```python
from build123d import *

# Parameters (mm, degrees)
BOSS_EXTRUDE1_DEPTH = 6
FILLET1_R           = 2
SKETCH2_R           = 1.5
CUT_EXTRUDE1_DEPTH  = 10
SKETCH3_W           = 6
SKETCH3_H           = 18.774257397
BOSS_EXTRUDE2_DEPTH = 2
FILLET2_R           = 10
SKETCH4_W           = 6
SKETCH4_H           = 2
BOSS_EXTRUDE3_DEPTH = 5
SKETCH5_W           = 6
SKETCH5_H           = 2
BOSS_EXTRUDE4_DEPTH = 7


with BuildPart() as part:
    # Sketch1 → Boss-Extrude1 (new body)
    with BuildSketch(Plane.XY):
        with BuildLine():
            Line((4.974937186, 0.5), (9.527119886, 0.5))
            Line((9.527119886, 0.5), (60, 0.5))
            Line((60, 0.5), (60, -40.25))
            Line((60, -40.25), (62, -40.25))
            Line((62, -40.25), (62, 4.331195296))
            Line((62, 4.331195296), (60, 4.331195296))
            Line((60, 4.331195296), (60, 2.5))
            Line((60, 2.5), (5.454356057, 2.5))
            ThreePointArc((5.454356057, 2.5), (-6, 0), (5.454356057, -2.5))
            Line((5.454356057, -2.5), (20, -2.5))
            Line((20, -2.5), (20, -0.5))
            Line((20, -0.5), (4.974937186, -0.5))
            Line((4.974937186, -0.5), (3.968626967, -0.5))
            ThreePointArc((3.968626967, -0.5), (-4, 0), (3.968626967, 0.5))
            Line((3.968626967, 0.5), (4.974937186, 0.5))
        make_face()
    extrude(amount=BOSS_EXTRUDE1_DEPTH)

    # Fillet1
    # the kernel refuses this fillet: 2 mm, written as the material it adds along each edge
    with BuildSketch(Plane(origin=(5.454356057, -2.5, 0), x_dir=(1, 0, 0), z_dir=(0, 0, 1))) as fillet1_piece_1:
        with BuildLine():
            CenterArc((1.16002222, -2), FILLET1_R, 90, 55.771133672)
            Line((-0.493572349, -0.875), (-0.52664424, -0.8525))
            ThreePointArc((-0.52664424, -0.8525), (-0.26328023, -0.428195989), (-0.036362374, 0.016666667))
            Line((-0.036362374, 0.016666667), (0, 0.04))
            Line((0, 0.04), (1.16002222, 0.04))
            Line((1.16002222, 0.04), (1.16002222, 0))
        make_face()
    extrude(amount=6)
    with BuildSketch(Plane(origin=(5.454356057, 2.5, 0), x_dir=(-0.491308051869414, 0.8709858771348026, 0), z_dir=(0, 0, 1))) as fillet1_piece_2:
        with BuildLine():
            CenterArc((1.172043497, -1.992979075), FILLET1_R, 94.802273988, 55.771133672)
            Line((-0.569928257, -1.010362971), (-0.604767692, -0.990710649))
            Line((-0.604767692, -0.990710649), (-0.034839435, 0.019652322))
            Line((-0.034839435, 0.019652322), (0.003348696, 0.039859581))
            ThreePointArc((0.003348696, 0.039859581), (0.502304356, 0.018937224), (1.001260016, 0.039859581))
            Line((1.001260016, 0.039859581), (1.004608712, 0))
        make_face()
    extrude(amount=6)
    with BuildSketch(Plane(origin=(60, 2.5, 0), x_dir=(-1, 0, 0), z_dir=(0, 0, 1))) as fillet1_piece_3:
        with BuildLine():
            CenterArc((1.992863511, -2), FILLET1_R, 90, 85.158341327)
            Line((0, -1.831195296), (-0.03985727, -1.827819202))
            ThreePointArc((-0.03985727, -1.827819202), (-0.04, -0.915597648), (-0.04, 0))
            Line((-0.04, 0), (0, 0.04))
            Line((0, 0.04), (1.992863511, 0.04))
            Line((1.992863511, 0.04), (1.992863511, 0))
        make_face()
    extrude(amount=6)
    with BuildSketch(Plane(origin=(60, 0.5, 0), x_dir=(-1, 0, 0), z_dir=(0, 0, 1))) as fillet1_piece_4:
        with BuildLine():
            CenterArc((FILLET1_R, FILLET1_R), FILLET1_R, 180, 90)
            Line((0, FILLET1_R), (-FILLET1_R * 0.02, FILLET1_R))
            Line((-FILLET1_R * 0.02, FILLET1_R), (-FILLET1_R * 0.02, -FILLET1_R * 0.02))
            Line((-FILLET1_R * 0.02, -FILLET1_R * 0.02), (FILLET1_R, -FILLET1_R * 0.02))
            Line((FILLET1_R, -FILLET1_R * 0.02), (FILLET1_R, 0))
        make_face()
    extrude(amount=6)

    # Sketch2 → Cut-Extrude1 (cut)
    with BuildSketch(Plane.XZ.offset(2.5)):
        with Locations((13.307189139, 3)):
            Circle(SKETCH2_R)
    extrude(amount=-CUT_EXTRUDE1_DEPTH, mode=Mode.SUBTRACT)

    # Sketch3 → Boss-Extrude2 (add)
    with BuildSketch(Plane(origin=(62, 0, 0), x_dir=(0, 0, -1), z_dir=(1, 0, 0))):
        with Locations((-3, -45.862871302)):
            Rectangle(SKETCH3_W, SKETCH3_H)
    extrude(amount=BOSS_EXTRUDE2_DEPTH)

    # Fillet2
    # the kernel refuses this fillet: 10 mm, written as the material it adds along each edge
    with BuildSketch(Plane(origin=(62, -36.475742603, 6), x_dir=(0, 1, 0), z_dir=(0, 0, -1))) as fillet2_piece_1:
        with BuildLine():
            CenterArc((6, 10), FILLET2_R, 233.130102354, 36.869897646)
            Line((0, 2), (-0.12, 1.84))
            ThreePointArc((-0.12, 1.84), (-0.2, 1), (-0.2, 0))
            Line((-0.2, 0), (0, -0.2))
            Line((0, -0.2), (6, -0.2))
            Line((6, -0.2), (6, 0))
        make_face()
    extrude(amount=6)

    # Sketch4 → Boss-Extrude3 (add)
    with BuildSketch(Plane.ZY.offset(-60)):
        with Locations((3, -39.25)):
            Rectangle(SKETCH4_W, SKETCH4_H)
    extrude(amount=BOSS_EXTRUDE3_DEPTH)

    # Sketch5 → Boss-Extrude4 (add)
    with BuildSketch(Plane.ZY.offset(-62)):
        with Locations((3, -54.25)):
            Rectangle(SKETCH5_W, SKETCH5_H)
    extrude(amount=BOSS_EXTRUDE4_DEPTH)


solid = part.part
```
The model under review builds one solid part; all positions refer to its coordinate system, in mm. A direction names the side the tool comes from. Give positions to 0.01 mm unless a question says otherwise; leave off trailing zeros. Write each loop counter-clockwise with the first axis right and the second up, starting at its lowest first coordinate (ties: lowest second). Pieces come first, ordered by that corner, then holes. Notation, with made-up numbers: M 68,-25 L 77,-25 A16 ccw 77,-9 Z; hole C 38.5,-0.5 d5. An arc over 180 degrees is marked long. Write item = value, one per line. Start each with the question number.
Q1. We need section A-A (z = 3). Give the number of separate pieces and of enclosed holes in the cut face, plus the area to 3 significant figures.
Q2. We need section B-B (x = 0). State the section outline as (y, z) points.
Q3. Mouldability with a two-part tool opening along Y and no side actions: class faces 5 (the face through (59, -53.25, 3)), 6 (the face through (64, -46, 3)), 7 (the face through (59, -40.25, 3)), 8 (the face through (59.34, 3.01, 2.96)) as released by +Y, released by -Y, zero draft, split by the parting line, or undercut.
Q4. For line 1 (X direction, y = -14.5, z = 4); line 2 (Y direction, x = 19, z = 0.45); line 3 (X direction, y = -44, z = 1.45), list the stretches that pass through material, from the lowest coordinate up.
Q5. Machinability: for faces 1 (the face through (58, -38.25, 3)), 2 (the face through (5.667, 2.739, 2.958)), 3 (the face through (55, -39, 3)), 4 (the face through (61, 4.331, 3)), which of the approach directions +Z, -Z, +X, -X, +Y, -Y give a long, thin tool a straight path to every point of the face, cutting with its end or side? Answer none if there is none.
Q6. We need section C-C (y = -46). State the section outline as (x, z) points.
Q7. We need section D-D (x = 30). State the section outline as (y, z) points.
Q8. Clearance check with flat-ended pins moving along their axes: pin 1 (1.8 mm diameter, centred on y = -16.5, z = 4.5, fed in from -X); pin 2 (2 mm diameter, centred on y = -39.5, z = 2, fed in from -X); pin 3 (1.8 mm diameter, centred on x = 25, z = 2.5, fed in from +Y). State where each tip first meets the part, or that it passes through.
Result set:
q1.separate_pieces = 3
q1.enclosed_holes = 0
q1.area = 342 mm2
q2.outline = M -6,0 L -4,0 L -4,6 L -6,6 Z; M 4,0 L 6,0 L 6,6 L 4,6 Z
q3.face_5 = undercut
q3.face_6 = zero draft
q3.face_7 = undercut
q3.face_8 = released by +Y
q4.line_1 = 60 to 62
q4.line_2 = -2.5 to -0.5, 0.5 to 2.5
q4.line_3 = 62 to 64
q5.face_1 = +Z, -Z, -X
q5.face_2 = +Z, -Z, +Y
q5.face_3 = +Z, -Z, -X, -Y
q5.face_4 = +Z, -Z, +X, +Y
q6.outline = M 62,0 L 64,0 L 64,6 L 62,6 Z
q7.outline = M 0.5,0 L 2.5,0 L 2.5,6 L 0.5,6 Z
q8.pin_1 = 60
q8.pin_2 = 55
q8.pin_3 = 2.5
